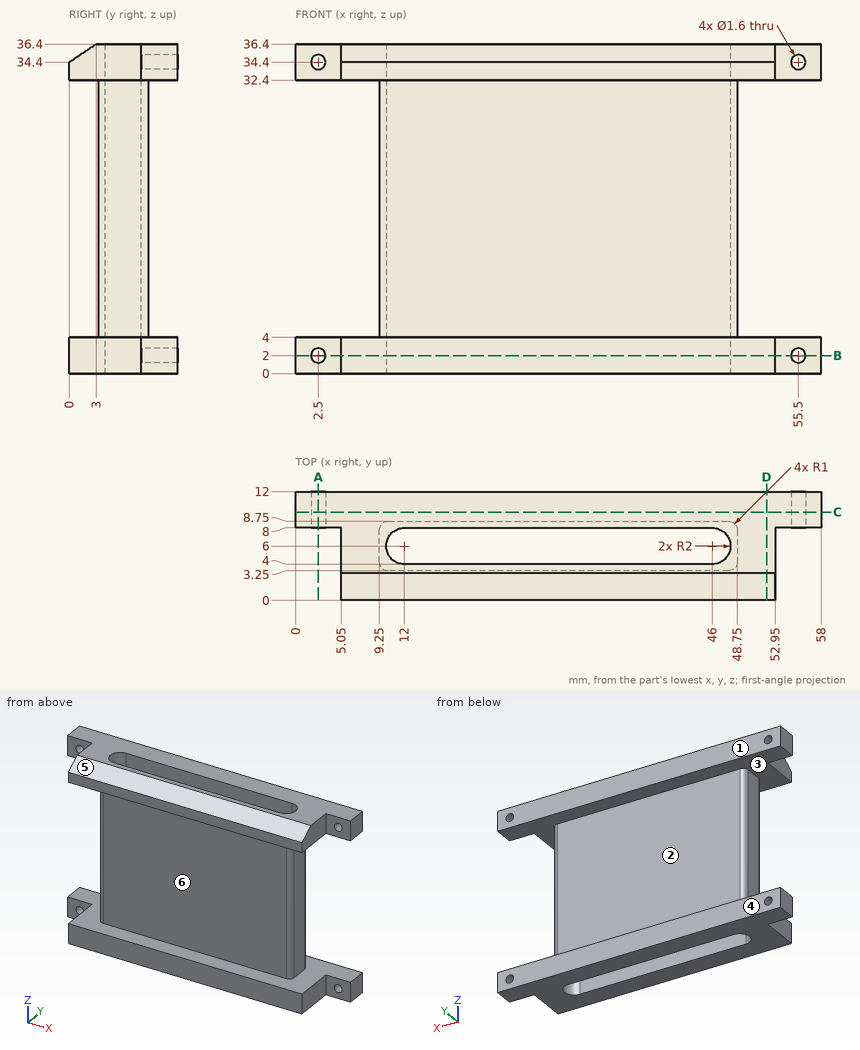
Check sheet for the drawn part. Datum: minimum x, y, z corner. Units: mm. A direction names the side the tool comes from. Round coordinates to 2 decimals unless told otherwise and drop trailing zeros. Order: outer loops, then holes, each group sorted by start corner. A loop starts at its lowest first (then second) coordinate and runs counter-clockwise, first axis right, second up. Notation, with made-up numbers: (80, -40) - (103, -40) arc R18 cw to (103, -27) - close; hole circle Ø11 at (72.25, 75). An arc over 180 degrees is marked (long way). Use a Markdown table: item, result. Add a question column.
(1) Depth check by flat-ended pin: pin 1 (1.8 mm diameter, centred on y = 5.5, z = 23.5, fed in from -X); pin 2 (8.5 mm diameter, centred on x = 30, z = 25, fed in from +Y); pin 3 (4.5 mm diameter, centred on y = 2.5, z = 34.5, fed in from -X); pin 4 (4.5 mm diameter, centred on x = 55, z = 35, fed in from -Y). Enter the tip coordinate at first touch or a pass-through.
(2) Sectioned sample at B-B, the plane z = 2. Enter the section's corners in (x, y), and give its area (3 significant figures).
(3) Sectioned sample at A-A, the plane x = 2.5. Enter the section's corners in (y, z), and give its area (3 significant figures).
(4) Material ranges on line 1 along X through (y, z) = (9.25, 2); line 2 along Y through (x, z) = (26, 23.5); line 3 along Z through (x, y) = (55.5, 9.7), recorded low to high. Write a range as [from, to].
(5) Sectioned sample at C-C, the plane y = 9.75. Enter the section's corners in (x, z), and give its area (3 significant figures).
(6) Sectioned sample at D-D, the plane x = 52. Enter the section's corners in (y, z).
(7) Tool access check on the marked faces 1 and 2. Record the directions out of +Z, -Z, +X, -X, +Y, -Y that give a thin tool (end or side, any length) a straight path to the whole face; none if there is none.
(8) Release check for a two-part mould opening along Z. For the marked faces 3, 4, 5 and 6 record: pulls with the +Z half, pulls with the -Z half, needs draft (parallel to the pull), parting line crosses it, or undercut.
Answers below:
| question | item | result |
|---|---|---|
| 1 | pin 1 | x = 9.25 |
| 1 | pin 2 | y = 8.75 |
| 1 | pin 3 | x = 5.05 |
| 1 | pin 4 | y = 0 |
| 2 | outline | (0, 8) - (1.7, 8) - (1.7, 12) - (0, 12) - close; (3.3, 8) - (5.05, 8) - (5.05, 0) - (52.95, 0) - (52.95, 8) - (54.7, 8) - (54.7, 12) - (3.3, 12) - close; (56.3, 8) - (58, 8) - (58, 12) - (56.3, 12) - close; hole (12, 4) - (46, 4) arc R2 ccw to (46, 8) - (12, 8) arc R2 ccw to start |
| 2 | area | 454 mm² |
| 3 | outline | (8, 0) - (12, 0) - (12, 1.2) - (8, 1.2) - close; (8, 2.8) - (12, 2.8) - (12, 4) - (8, 4) - close; (8, 32.4) - (12, 32.4) - (12, 33.6) - (8, 33.6) - close; (8, 35.2) - (12, 35.2) - (12, 36.4) - (8, 36.4) - close |
| 3 | area | 19.2 mm² |
| 4 | line 1 | [0, 1.7], [3.3, 54.7], [56.3, 58] |
| 4 | line 2 | [3.25, 4], [8, 8.75] |
| 4 | line 3 | [0, 1.2], [2.8, 4], [32.4, 33.6], [35.2, 36.4] |
| 5 | outline | (0, 0) - (58, 0) - (58, 4) - (0, 4) - close; (0, 32.4) - (58, 32.4) - (58, 36.4) - (0, 36.4) - close; hole circle Ø1.6 at (2.5, 2); hole circle Ø1.6 at (2.5, 34.4); hole circle Ø1.6 at (55.5, 2); hole circle Ø1.6 at (55.5, 34.4) |
| 5 | area | 456 mm² |
| 6 | outline | (0, 0) - (12, 0) - (12, 4) - (0, 4) - close; (0, 32.4) - (12, 32.4) - (12, 36.4) - (3, 36.4) - (0, 34.4) - close |
| 7 | face 1 | +Z, -Z, +X, -X, +Y |
| 7 | face 2 | +X, -X, +Y |
| 8 | face 3 | undercut |
| 8 | face 4 | needs draft |
| 8 | face 5 | pulls with the +Z half |
| 8 | face 6 | undercut |
